Geometry check sheet. Reference: the model listing, model coordinates, mm. A direction names the side the tool comes from. Round coordinates to 2 decimals unless told otherwise and drop trailing zeros. Order: outer loops, then holes, each group sorted by start corner. A loop starts at its lowest first (then second) coordinate and runs counter-clockwise, first axis right, second up. Notation, with made-up numbers: (49.5, 75.25) - (103.5, 75.25) arc R18 ccw to (103.5, 102.25) - close; hole circle Ø8 at (-20, 15.5). An arc over 180 degrees is marked (long way). Write each question's results on one line, items separated by ' | '.
```python
from build123d import *

# Parameters (mm, degrees)
F0_W     = 5
F0_H     = 18
F1_DEPTH = 20
F2_SIZE  = 0.99999
F3_W     = 4.7912499867
F3_H     = 21.5901492629
F4_DEPTH = 5


# Not quite as in the source:
# - a fillet or chamfer is up to 0.001 mm smaller than in the source, because OpenCascade refuses the exact size


with BuildPart() as f1:
    # F0 (on Top) → F1 (new body)
    with BuildSketch(Plane.XY):
        Polygon((-2.3178061422, 7.6096997074), (-7.9299724714, 7.6096997074), (-8.6440549978, 6.9096381776), (-8.6440549978, -11.3519806733), (-8.0234205974, -12.1360807569), (-2.2334722516, -12.1360807569), (-1.6440549978, -11.3282519997), (-1.6440549978, 6.8707413895), align=None)
        with Locations((-5.1440549978, -2.3903002926)):
            Rectangle(F0_W, F0_H, mode=Mode.SUBTRACT)
    extrude(amount=F1_DEPTH)

    # F2 (size 1 in the source; OpenCascade refuses exactly that, so slightly less here)
    f2_edges = [f1.edges().sort_by_distance(p)[0] for p in [
        (-8.644055, -2.221171, 20),
        (-8.644055, -2.221171, 0),
        (-1.644055, -2.228755, 0),
        (-1.644055, -2.228755, 20),
    ]]
    chamfer(f2_edges, length=F2_SIZE)

    # F3 (on face) → F4 (cut)
    with BuildSketch(Plane(origin=(-8.6440549978, 0, 0), x_dir=(0, -1, 0), z_dir=(-1, 0, 0))):
        with Locations((2.3956249934, 9.8618984921)):
            Rectangle(F3_W, F3_H)
    extrude(amount=-F4_DEPTH, mode=Mode.SUBTRACT)


solid = f1.part
```
(1) Material ranges on line 1 (X direction, y = 4.75, z = 15.5); line 2 (Y direction, x = -6.75, z = 3.75); line 3 (X direction, y = -4.75, z = 7), recorded low to high.
Answers follow:
line 1: -8.64 to -7.64, -2.64 to -1.64 | line 2: -12.14 to -11.39, 6.61 to 7.61 | line 3: -2.64 to -1.64
(2) Section check A-A (x = -3.25). Record the cut outline in (y, z).
Answers follow:
outline: (-12.14, 0) - (-11.39, 0) - (-11.39, 20) - (-12.14, 20) - close; (6.61, 0) - (7.61, 0) - (7.61, 20) - (6.61, 20) - close
(3) Section check C-C (z = 13.5). Record the cut outline in (x, y).
Answers follow:
outline: (-8.64, -11.35) - (-8.02, -12.14) - (-2.23, -12.14) - (-1.64, -11.33) - (-1.64, 6.87) - (-2.32, 7.61) - (-7.93, 7.61) - (-8.64, 6.91) - (-8.64, 0) - (-7.64, 0) - (-7.64, 6.61) - (-2.64, 6.61) - (-2.64, -11.39) - (-7.64, -11.39) - (-7.64, -4.79) - (-8.64, -4.79) - close
(4) Draft check along X on faces 1 (the face through (-2.644, -3, 10)), 2 (the face through (-8, 0, 10)), 3 (the face through (-1.943, -11.738, 9.866)), 4 (the face through (-8.137, 3.858, 0.493)). Enter one of: released by +X, released by -X, zero draft, split by the parting line, or undercut.
Answers follow:
face 1: undercut | face 2: zero draft | face 3: released by +X | face 4: released by -X
(5) Access from +Z, -Z, +X, -X, +Y, -Y to the whole of each face (thin tool, end or side, straight path). Record for faces 5 (the face through (-8.137, 3.858, 19.507)), 6 (the face through (-5, -11.39, 10)), 7 (the face through (-8, -4.791, 10)).
Answers follow:
face 5: +Z, -X, +Y, -Y | face 6: +Z, -Z | face 7: +Z, -Z, -X
